Here's the drawing with two shaded views (mm, measured from the low corner). I have some questions. Give positions to 0.01 mm unless a question says otherwise; leave off trailing zeros. Loops run counter-clockwise (first coordinate to the right, second up) from the corner with the lowest first, then second, coordinate; pieces in that order, holes last. Notation, with made-up numbers: (17.5, -15.5) - (31.5, -15.5) arc R13 cw to (31.5, 1.5) - close; hole circle Ø1 at (-32.5, 78). An arc over 180 degrees is marked (long way). Answer as a JSON object with one key per item and string values. Group by question number.
Item 1: Will these pins go through, and if not, where does the flat tip stop? pin 1 (8 mm diameter, centred on x = 131, y = 62.5, fed in from +Z); pin 2 (4 mm diameter, centred on y = 115.5, z = 8, fed in from +X); pin 3 (2 mm diameter, centred on x = 90.5, y = 31.5, fed in from -Z).
Item 2: Thinking about a two-plate mould opening in Y: for the marked faces 1, 2 and 3, which applies, pulls with the +Y half, pulls with the -Y half, needs draft (parallel to the pull), parting line crosses it, or undercut?
Item 3: Suppose I cut it at A-A on z = 8.5. Write out the boundary of the cut face in (x, y).
Item 4: Suppose I cut it at D-D on y = 19.5. Write out the boundary of the cut face in (x, z).
Item 5: Please list where these lines run through material, in increasing order: L1, parallel to Y at x = 105, z = 11; L2, parallel to Z at x = 12, y = 87; L3, parallel to X at y = 143, z = 6.5.
Item 6: Suppose I cut it at C-C on y = 148. Write out the boundary of the cut face in (x, z).
Item 7: Suppose I cut it at B-B on x = 44. Write out the boundary of the cut face in (y, z).
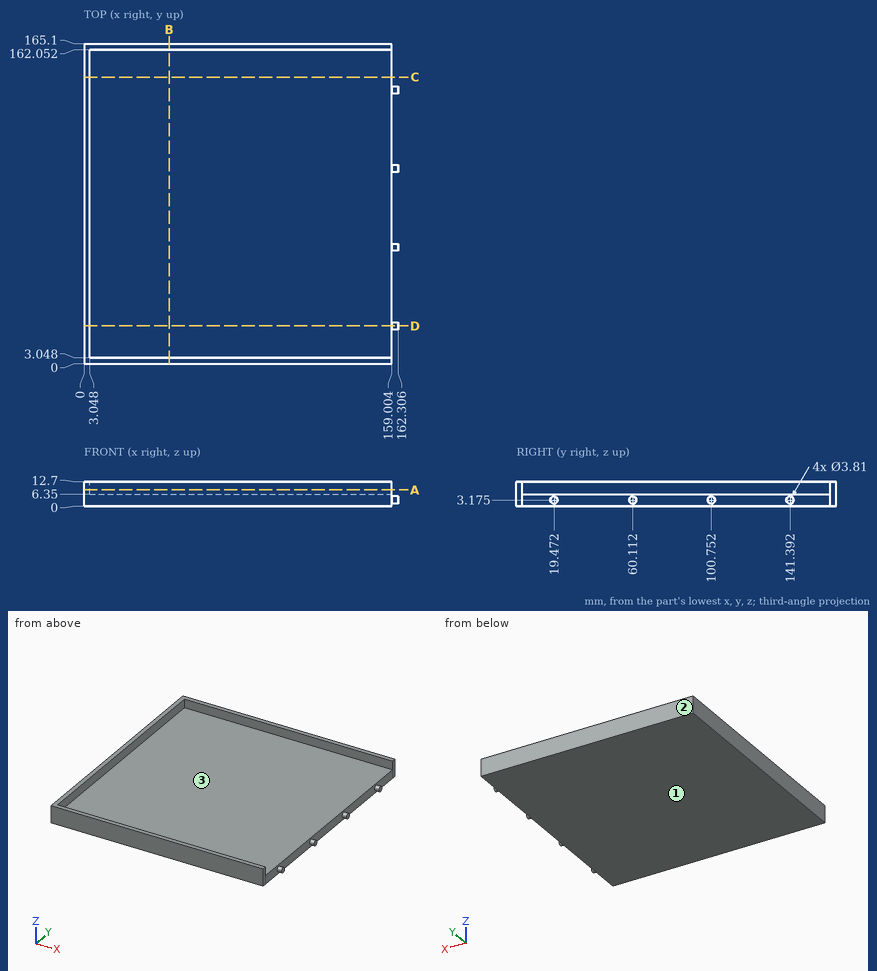
Worked out:
{
 "1": {"pin 1": "stops at z = 6.35", "pin 2": "stops at x = 159", "pin 3": "stops at z = 0"},
 "2": {"face 1": "needs draft", "face 2": "pulls with the +Y half", "face 3": "undercut"},
 "3": {"outline": "(0, 0) - (159, 0) - (159, 3.05) - (3.05, 3.05) - (3.05, 162.05) - (159, 162.05) - (159, 165.1) - (0, 165.1) - close"},
 "4": {"outline": "(0, 0) - (159, 0) - (159, 1.27) - (162.31, 1.27) - (162.31, 5.08) - (159, 5.08) - (159, 6.35) - (3.05, 6.35) - (3.05, 12.7) - (0, 12.7) - close"},
 "5": {"L1": "y = 0 to 3.05, 162.05 to 165.1", "L2": "z = 0 to 6.35", "L3": "x = 0 to 3.05"},
 "6": {"outline": "(0, 0) - (159, 0) - (159, 6.35) - (3.05, 6.35) - (3.05, 12.7) - (0, 12.7) - close"},
 "7": {"outline": "(0, 0) - (165.1, 0) - (165.1, 12.7) - (162.05, 12.7) - (162.05, 6.35) - (3.05, 6.35) - (3.05, 12.7) - (0, 12.7) - close"}
}
